Job drawing, mm, ordinate dimensions from the low corner. One solid piece. Give positions to 0.01 mm unless a question says otherwise; leave off trailing zeros. Order: outer loops, then holes, each group sorted by start corner. A loop starts at its lowest first (then second) coordinate and runs counter-clockwise, first axis right, second up.
1. Slice it at D-D on y = 1.2. Give the number of separate pieces and of enclosed holes in the cut face, and give its area (3 significant figures).
2. Slice it at A-A on z = 19. List the corners of the cut face in (x, y).
3. Slice it at C-C on x = 48. List the corners of the cut face in (y, z), and give its area (3 significant figures).
4. Drop a flat-ended pin along its axis: pin 1 Ø1.5 at (y, z) = (0.5, 22) entering from -X. Give the stop position or say it passes through.
5. Slice it at B-B on x = 62. List the corners of the cut face in (y, z), and give its area (3 significant figures).
6. Probe line 1 (X direction, y = 1.7, z = 19); line 2 (X direction, y = 0.3, z = 42); line 3 (Z direction, x = 67, y = 0.95). List the from-to ranges inside material, lowest first.
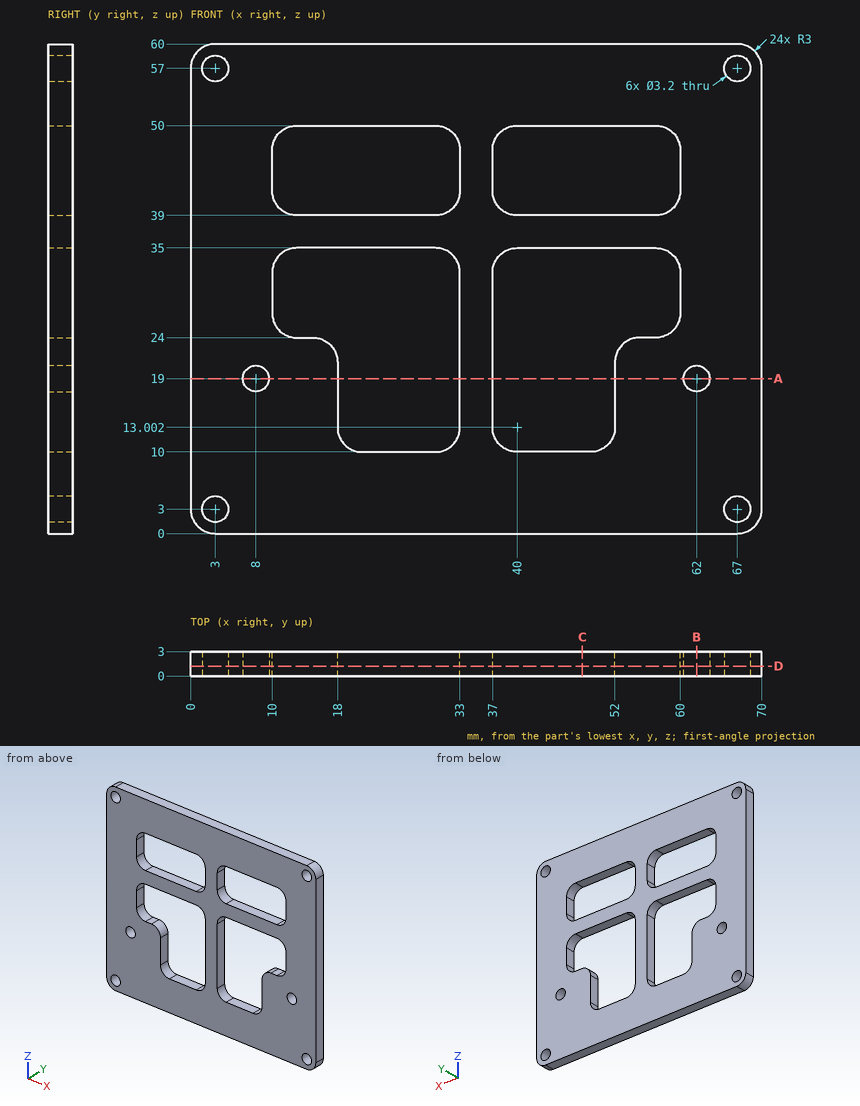
Data:
1. separate pieces: 1
1. enclosed holes: 10
1. area: 2,740 mm2
2. outline: (0, 0) - (6.4, 0) - (6.4, 3) - (0, 3) - close; (9.6, 0) - (18, 0) - (18, 3) - (9.6, 3) - close; (33, 0) - (37, 0) - (37, 3) - (33, 3) - close; (52, 0) - (60.4, 0) - (60.4, 3) - (52, 3) - close; (63.6, 0) - (70, 0) - (70, 3) - (63.6, 3) - close
3. outline: (0, 0) - (3, 0) - (3, 10) - (0, 10) - close; (0, 35) - (3, 35) - (3, 39) - (0, 39) - close; (0, 50) - (3, 50) - (3, 60) - (0, 60) - close
3. area: 72.0 mm2
4. pin 1: stops at x = 0
5. outline: (0, 0) - (3, 0) - (3, 17.4) - (0, 17.4) - close; (0, 20.6) - (3, 20.6) - (3, 60) - (0, 60) - close
5. area: 170 mm2
6. line 1: x = 0 to 6.4, 9.6 to 18, 33 to 37, 52 to 60.4, 63.6 to 70
6. line 2: x = 0 to 10, 33 to 37, 60 to 70
6. line 3: z = 0 to 1.4, 4.6 to 55.4, 58.6 to 60
